Geometry check sheet. Reference: the model listing, model coordinates, mm. A direction names the side the tool comes from. Round coordinates to 2 decimals unless told otherwise and drop trailing zeros. Loops run counter-clockwise (first coordinate to the right, second up) from the corner with the lowest first, then second, coordinate; pieces in that order, holes last. Notation, with made-up numbers: (-14, -1) -> (8, -1) arc R14 ccw to (8, 9) -> close; hole circle Ø6 at (67.25, -9). An arc over 180 degrees is marked (long way). Use a Markdown table: item, result. Add a question column.
Q1. Release check for a two-part mould opening along Z. For faces 1 (the face through (0, 5, 0)), 2 (the face through (24.65, 5.722, 43.503)), 3 (the face through (-24.65, 5.722, -43.503)) record: released by +Z, released by -Z, zero draft, split by the parting line, or undercut.
Q2. Material ranges on L1, parallel to Z at x = 21.5, y = 2.5; L2, parallel to Z at x = -16, y = 2; L3, parallel to X at y = 0.5, z = 7, recorded low to high.
Q3. Sectioned sample at B-B, the plane x = -37. Enter the section's corners in (y, z), then the cut area to 3 significant figures.
Q4. Sectioned sample at D-D, the plane z = -15.5. Enter the section's corners in (x, y).
Q5. Gauge pin test, flat ends, axial feed: P1, Ø1.5, axis at x = -34.5, y = 1.5, coming from the +Z side; P2, Ø3, axis at x = 40, y = 3.5, coming from the +Z side; P3, Ø4, axis at x = 16.5, y = 3, coming from the +Z side. Record the tip position at first contact, or that the pin passes through.
Q6. Sectioned sample at A-A, the plane y = 2.75. Enter the section's corners in (x, z).
Q7. Set-up check for faces 4 (the face through (-33, 0, -18)), 5 (the face through (-28, 2, 2.7)), 6 (the face through (11.49, 2.46, 25.3)): record each of +Z, -Z, +X, -X, +Y, -Y from which the full face is reachable in a straight line by a thin tool's end or side.
Q8. Sectioned sample at C-C, the plane z = 40. Enter the section's corners in (x, y).
```python
from build123d import *

# Parameters (mm, degrees)
BOSS_EXTRUDE1_DEPTH     = 8
SKETCH2_W               = 100
SKETCH2_H               = 5.4
CUT_EXTRUDE_THIN1_DEPTH = 5


with BuildPart() as part:
    # Sketch1 → Boss-Extrude1 (new body)
    with BuildSketch(Plane(origin=(0, 0, 0), x_dir=(1, 0, 0), z_dir=(0, 1, 0))):
        Polygon((0, 57.735026919), (-50, 28.867513459), (-50, -28.867513459), (0, -57.735026919), (50, -28.867513459), (50, 28.867513459), align=None)
    extrude(amount=BOSS_EXTRUDE1_DEPTH)

    # Sketch2 → Cut-Extrude-Thin1 (cut)
    with BuildSketch(Plane.XZ):
        Polygon((-27.33826859, 41.951270189), (22.66173141, -44.651270189), (27.33826859, -41.951270189), (-22.66173141, 44.651270189), align=None)
        Polygon((22.66173141, 44.651270189), (-27.33826859, -41.951270189), (-22.66173141, -44.651270189), (27.33826859, 41.951270189), align=None)
        Rectangle(SKETCH2_W, SKETCH2_H)
    extrude(amount=-CUT_EXTRUDE_THIN1_DEPTH, mode=Mode.SUBTRACT)


solid = part.part
```
Values:
| question | item | result |
|---|---|---|
| 1 | face 1 | undercut |
| 1 | face 2 | released by +Z |
| 1 | face 3 | released by -Z |
| 2 | L1 | -45.32 to -42.64, -31.84 to -2.7, 2.7 to 31.84, 42.64 to 45.32 |
| 2 | L2 | -48.5 to -33.11, -22.31 to -2.7, 2.7 to 22.31, 33.11 to 48.5 |
| 2 | L3 | -50 to -7.16, -0.92 to 0.92, 7.16 to 50 |
| 3 | outline | (0, -36.37) -> (8, -36.37) -> (8, 36.37) -> (0, 36.37) -> (0, 2.7) -> (5, 2.7) -> (5, -2.7) -> (0, -2.7) -> close |
| 3 | area | 555 mm^2 |
| 4 | outline | (-50, 0) -> (-12.07, 0) -> (-12.07, 5) -> (-5.83, 5) -> (-5.83, 0) -> (5.83, 0) -> (5.83, 5) -> (12.07, 5) -> (12.07, 0) -> (50, 0) -> (50, 8) -> (-50, 8) -> close |
| 5 | P1 | z = 38.25 |
| 5 | P2 | z = 35.51 |
| 5 | P3 | z = 49.36 |
| 6 | outline | (-50, -28.87) -> (-27.34, -41.95) -> (-4.68, -2.7) -> (-50, -2.7) -> close; (-50, 2.7) -> (-4.68, 2.7) -> (-27.34, 41.95) -> (-50, 28.87) -> close; (-22.66, -44.65) -> (0, -57.74) -> (22.66, -44.65) -> (0, -5.4) -> close; (-22.66, 44.65) -> (0, 5.4) -> (22.66, 44.65) -> (0, 57.74) -> close; (4.68, -2.7) -> (27.34, -41.95) -> (50, -28.87) -> (50, -2.7) -> close; (4.68, 2.7) -> (50, 2.7) -> (50, 28.87) -> (27.34, 41.95) -> close |
| 7 | face 4 | +Z, -Z, +X, -X, -Y |
| 7 | face 5 | +X, -X, -Y |
| 7 | face 6 | -Y |
| 8 | outline | (-30.72, 0) -> (-26.21, 0) -> (-26.21, 5) -> (-19.98, 5) -> (-19.98, 0) -> (19.98, 0) -> (19.98, 5) -> (26.21, 5) -> (26.21, 0) -> (30.72, 0) -> (30.72, 8) -> (-30.72, 8) -> close |
